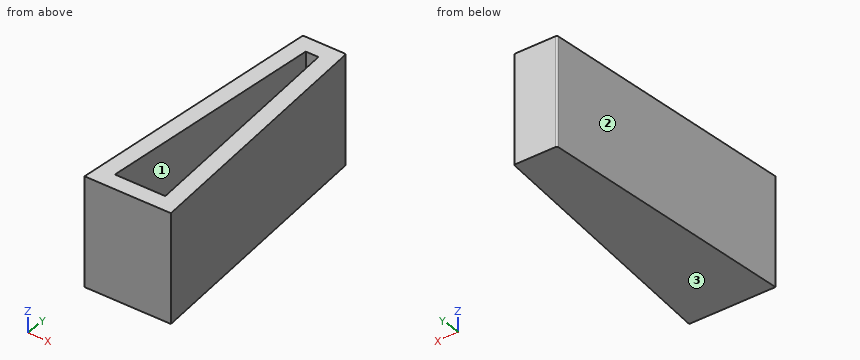
from build123d import *

# Parameters (mm, degrees)
F1_DEPTH = 15
F2_T     = -2.3


with BuildPart() as f1:
    # F0 (on Top) → F1 (new body)
    with BuildSketch(Plane.XY):
        with BuildLine():
            Line((2.815764, 36.5), (0, 36.5))
            Line((0, 36.5), (-2.789257, 36.5))
            ThreePointArc((-2.789257, 36.5), (-2.944258, 36.439489), (-3.017263, 36.289965))
            Line((-3.017263, 36.289965), (-6, 0))
            Line((-6, 0), (0, 0))
            Line((0, 0), (6, 0))
            Line((6, 0), (3.015092, 36.316383))
            ThreePointArc((3.015092, 36.316383), (2.951269, 36.4471), (2.815764, 36.5))
        make_face()
    extrude(amount=F1_DEPTH)

    # F2
    f2_openings = [f1.faces().sort_by_distance(p)[0] for p in [
        (2e-05, 16.221217, 15),
    ]]
    offset(amount=F2_T, openings=f2_openings)


solid = f1.part
Design review of the part built by this model. Coordinates are the model's own, in mm. Face numbers are marked on the shaded views. Give positions to 0.01 mm unless a question says otherwise; leave off trailing zeros. Loops run counter-clockwise (first coordinate to the right, second up) from the corner with the lowest first, then second, coordinate; pieces in that order, holes last. Notation, with made-up numbers: (88, 63) - (118, 63) arc R34 cw to (118, 99) - close; hole circle Ø9 at (47, 5.25). An arc over 180 degrees is marked (long way). Use CSV: the item, a comma, the result in double quotes. Start each with the question number.
1. Add section A-A (x = 0). State the section outline as (y, z) points.
2. Insertion check: P1, Ø5, axis at y = 9, z = 8.5, coming from the +X side; P2, Ø4, axis at y = 15.5, z = 2.5, coming from the -X side; P3, Ø2, axis at y = 5, z = 4, coming from the +X side. Each pin has a flat end and moves straight along its axis. Give the tip position at first contact, or say it passes through.
3. Add section C-C (y = 22). State the section outline as (x, z) points, plus the area to 3 significant figures.
4. Draft analysis for pull direction X (two halves, no side actions). For the marked faces 1, 2 and 3, state which applies: released by +X, released by -X, zero draft, split by the parting line, or undercut.
5. Add section B-B (z = 12.75). State the section outline as (x, y) points, plus the area to 3 significant figures.
6. Add section D-D (x = 5). State the section outline as (y, z) points, plus the area to 4 significant figures.
7. Wall thickness on L1, parallel to Y at x = -0.25, z = 7; L2, parallel to X at y = 7, z = 13.25; L3, parallel to X at y = 10, z = 11.75: over which ranges is each line inside the solid? List them lowest first.
Results found:
1,outline,"(0, 0) - (36.5, 0) - (36.5, 15) - (34.2, 15) - (34.2, 2.3) - (2.3, 2.3) - (2.3, 15) - (0, 15) - close"
2,P1,"stops at x = 5.47"
2,P2,"stops at x = -4.89"
2,P3,"stops at x = 5.67"
3,outline,"(-4.19, 0) - (4.19, 0) - (4.19, 15) - (1.88, 15) - (1.88, 2.3) - (-1.88, 2.3) - (-1.88, 15) - (-4.19, 15) - close"
3,area,"77.9 mm²"
4,face 1,"undercut"
4,face 2,"released by -X"
4,face 3,"zero draft"
5,outline,"(-6, 0) - (6, 0) - (3.02, 36.32) arc R0.2 ccw to (2.82, 36.5) - (-2.79, 36.5) arc R0.23 ccw to (-3.02, 36.29) - close; hole (-3.5, 2.3) - (3.5, 2.3) - (0.88, 34.2) - (-0.88, 34.2) - close"
5,area,"189 mm²"
6,outline,"(0, 0) - (12.17, 0) - (12.17, 15) - (0, 15) - close"
6,area,"182.5 mm²"
7,L1,"y = 0 to 2.3, 34.2 to 36.5"
7,L2,"x = -5.42 to -3.12, 3.12 to 5.42"
7,L3,"x = -5.18 to -2.87, 2.87 to 5.18"
